Solid Edge part; units mm, degrees
sketch "Sketch1" plane through (0, 0, 0) normal (0, 0, 1) x (1, 0, 0)
  line L0 (-15.0761, 2.2218) -> (-15.0761, 52.2218)
  line L1 (-15.0761, 52.2218) -> (-57.5761, 52.2218)
  line L2 (-57.5761, 52.2218) -> (-57.5761, 2.2218)
  line L3 (-57.5761, 2.2218) -> (-15.0761, 2.2218)
  line L4 (-25.0761, 30.4218) -> (-25.0761, 42.2218)
  line L5 (-25.0761, 42.2218) -> (-47.5761, 42.2218)
  line L6 (-47.5761, 42.2218) -> (-47.5761, 30.4218)
  line L7 (-47.5761, 30.4218) -> (-25.0761, 30.4218)
extrude "Protrusion1" add sketch "Sketch1" against normal blind 10
sketch "Sketch2" plane through (0, 0, 0) normal (0, 0, 1) x (1, 0, 0)
  line L0 (-23.2755, 17.1218) -> (-23.2755, 22.0207)
  line L1 (-23.2755, 22.0207) -> (-32.5481, 22.0207)
  line L2 (-32.5481, 22.0207) -> (-32.5481, 17.1218)
  line L3 (-32.5481, 17.1218) -> (-23.2755, 17.1218)
  line L4 (-23.2755, 7.1218) -> (-23.2755, 2.2218)
  line L5 (-23.2755, 2.2218) -> (-32.5481, 2.2218)
  line L6 (-32.5481, 2.2218) -> (-32.5481, 7.1218)
  line L7 (-32.5481, 7.1218) -> (-23.2755, 7.1218)
extrude "ExtrudedProtrusion_3" add sketch "Sketch2" along normal blind 6
sketch "Sketch3" plane through (-27.9118, 22.0207, 3) normal (0, 1, 0) x (1, 0, 0)
  circle A0 centre (0, 0) radius 1.55
extrude "ExtrudedCutout_1" cut sketch "Sketch3" against normal blind 17.5849
sketch "Sketch4" plane through (0, 0, 0) normal (0, 0, 1) x (1, 0, 0)
  circle A0 centre (-27.9118, 12.1218) radius 61.5
extrude "ExtrudedProtrusion_4" add sketch "Sketch4" against normal blind 10
sketch "Sketch5" plane through (0, 0, 0) normal (0, 0, 1) x (1, 0, 0)
  line L0 (-47.5761, 42.2218) -> (-47.5761, 30.4218)
  line L1 (-47.5761, 30.4218) -> (-25.0761, 30.4218)
  line L2 (-25.0761, 30.4218) -> (-25.0761, 42.2218)
  line L3 (-25.0761, 42.2218) -> (-47.5761, 42.2218)
extrude "ExtrudedCutout_2" cut sketch "Sketch5" against normal blind 44.8908
sketch "Sketch6" plane through (-27.9118, 12.1218, -5) normal (0, 0, -1) x (0, 1, 0)
  circle A0 centre (0, 0) radius 60.5
  circle A1 centre (0, 0) radius 63
extrude "ExtrudedProtrusion_6" add sketch "Sketch6" along normal blind 20
sketch "Sketch7" plane through (-27.9118, -50.8782, -15) normal (0, -1, 0) x (0, 0, 1)
  line L0 (-7.0569, 27.7607) -> (2.0569, 27.7607)
  line L1 (2.0569, 27.7607) -> (2.0569, -27.7607)
  line L2 (2.0569, -27.7607) -> (-7.0569, -27.7607)
  line L3 (-7.0569, -27.7607) -> (-7.0569, 27.7607)
extrude "ExtrudedCutout_3" cut sketch "Sketch7" against normal blind 172.1374
pattern_circular "Pattern_1" count 4 over 360 about axis through (-27.9118, 12.1218, -25) along (0, 0, 1) of "ExtrudedCutout_3"
sketch "Sketch8" plane through (-27.9118, 12.1218, 0) normal (0, 0, 1) x (0, -1, 0)
  circle A0 centre (0, 0) radius 59.5
  circle A1 centre (0, 0) radius 61.5
extrude "Protrusion2" add sketch "Sketch8" along normal blind 6
fillet "Round_1" radius 2.75 4 edges at (-32.5481, 4.6718, 6) (-23.2755, 4.6718, 6) (-32.5481, 19.5713, 6) (-23.2755, 19.5713, 6)
sketch "Sketch9" plane through (-27.9118, 12.1218, 0) normal (0, 0, 1) x (1, 0, 0)
  circle A0 centre (-22.0643, 24.2) radius 1.15
  circle A1 centre (5.2357, 24.2) radius 1.15
extrude "Cutout4" cut sketch "Sketch9" along normal mid plane 85.0753
sketch "Sketch10" plane through (-27.9118, 12.1218, 0) normal (0, 0, 1) x (1, 0, 0)
  circle A0 centre (-25, 0) radius 1.65
  circle A1 centre (25, 0) radius 1.65
extrude "ExtrudedCutout_8" cut sketch "Sketch10" along normal mid plane 174.1948
Work out the finished part from the listing and answer in its coordinate system (mm). A direction names the side the tool comes from. Coordinates: 2 decimals unless noted, no trailing zeros. Write each loop counter-clockwise with the first axis right and the second up, starting at its lowest first coordinate (ties: lowest second). Pieces come first, ordered by that corner, then holes. Notation, with made-up numbers: (-28, 7) - (-23, 7) arc R19 ccw to (-23, 21) - close; hole circle Ø7 at (36.5, -13.5). An arc over 180 degrees is marked (long way). One line per question, with ' | ' between items.
1) Find section C-C, the plane z = -6.5. Determine the outline of the cut face in (x, y), and give its area (3 significant figures).
Checks:
outline: circle Ø126 at (-27.91, 12.12); hole circle Ø3.3 at (-52.91, 12.12); hole circle Ø2.3 at (-49.98, 36.32); hole (-47.58, 30.42) - (-25.08, 30.42) - (-25.08, 42.22) - (-47.58, 42.22) - close; hole circle Ø2.3 at (-22.68, 36.32); hole circle Ø3.3 at (-2.91, 12.12) | area: 12,200 mm2
2) Flat-ended cylindrical pins translate along their axes: P1, Ø12, axis at y = -22, z = 1.5, coming from the +X side; P2, Ø1.6, axis at y = 18.5, z = 1, coming from the +X side; P3, Ø5, axis at x = 12, z = -15, coming from the -Y side. Find the tip coordinate at first contact, or state that the pin passes through.
Checks:
P1: x = 26.78 | P2: x = 33.33 | P3: y = -38.57
3) Find section A-A, the plane x = -34. Determine the outline of the cut face in (y, z), and give its area (3 significant figures).
Checks:
outline: (-50.58, -25) - (-48.07, -25) - (-48.07, -22.06) - (-50.58, -22.06) - close; (-50.58, -12.94) - (-48.07, -12.94) - (-48.07, -10) - (30.42, -10) - (30.42, 0) - (-47.07, 0) - (-47.07, 6) - (-49.08, 6) - (-49.08, -5) - (-50.58, -5) - close; (42.22, -10) - (72.31, -10) - (72.31, -12.94) - (74.83, -12.94) - (74.83, -5) - (73.32, -5) - (73.32, 6) - (71.31, 6) - (71.31, 0) - (42.22, 0) - close; (72.31, -25) - (74.83, -25) - (74.83, -22.06) - (72.31, -22.06) - close | area: 1,170 mm2
4) Consider probe 1 along Y at (x, z) = (-29, 5); probe 2 along X at (y, z) = (6.1, 3); probe 3 along Z at (x, y) = (-47.5, 2.5). Determine where each line is inside the solid, lowest interval first. Write a range as [from, to].
Checks:
probe 1: [-49.37, -47.37], [2.22, 7.12], [17.12, 22.02], [71.61, 73.61] | probe 2: [-89.12, -87.11], [-32.55, -29.46], [-26.36, -23.28], [31.28, 33.29] | probe 3: [-10, 0]
5) Find section D-D, the plane y = 57.5. Determine the outline of the cut face in (x, z).
Checks:
outline: (-71.61, -25) - (-67.93, -25) - (-67.93, -10) - (12.1, -10) - (12.1, -25) - (15.79, -25) - (15.79, -5) - (13.6, -5) - (13.6, 6) - (10.57, 6) - (10.57, 0) - (-66.4, 0) - (-66.4, 6) - (-69.42, 6) - (-69.42, -5) - (-71.61, -5) - close
6) The mould has two halves that part along Z. Classify faces 1 (the face through (-28, 20, 6)), 2 (the face through (-28, -49, -12.943)), 3 (the face through (-47.576, 36, -5)), 4 (the face through (-0.151, 67, -17)): +Z half, -Z half, draft (parallel to the pull), parting line (faces both ways), or undercut.
Checks:
face 1: +Z half | face 2: undercut | face 3: draft | face 4: undercut
7) For faces 5 (the face through (-83, 39.882, -17)), 6 (the face through (-29.46, 19.61, 2.93)), 7 (the face through (-0.151, -43, -17)), determine the directions among +Z, -Z, +X, -X, +Y, -Y from which every point of the face is accessible in a straight line to the end or side of a thin tool.
Checks:
face 5: +X, -X | face 6: none | face 7: +Y, -Y
